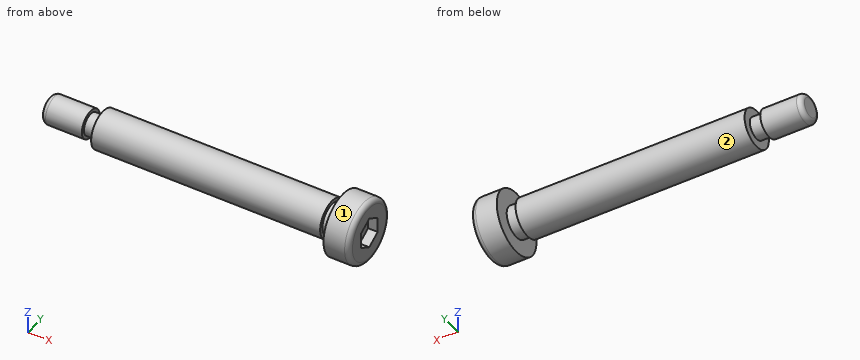
```python
from build123d import *

# Parameters (mm, degrees)
CUT_EXTRUDE1_DEPTH = 2


with BuildPart() as part:
    # Sketch2 → Revolve1 (revolve)
    with BuildSketch(Plane.XY):
        with BuildLine():
            Line((-50, 3.97), (-2.3, 3.97))
            Line((-2.3, 3.97), (-2.3, 3.25))
            Line((-2.3, 3.25), (0, 3.25))
            Line((0, 3.25), (0, 6.5))
            Line((0, 6.5), (4.4, 6.5))
            ThreePointArc((4.4, 6.5), (5.107106781, 6.207106781), (5.4, 5.5))
            Line((5.4, 5.5), (5.4, 0))
            Line((5.4, 0), (-61.15, 0))
            Line((-61.15, 0), (-61.15, 1.925))
            ThreePointArc((-61.15, 1.925), (-60.857106781, 2.632106781), (-60.15, 2.925))
            Line((-60.15, 2.925), (-52.6, 2.925))
            Line((-52.6, 2.925), (-52.6, 2.25))
            Line((-52.6, 2.25), (-50, 2.25))
            Line((-50, 2.25), (-50, 3.97))
        make_face()
    revolve(axis=Axis((-61.15, 0, 0), (1, 0, 0)))

    # Sketch3 → Cut-Extrude1 (cut)
    with BuildSketch(Plane(origin=(5.4, 0, 0), x_dir=(0, 0, -1), z_dir=(1, 0, 0))):
        Polygon((1.58771324, 2.75), (-1.58771324, 2.75), (-3.175426481, 0), (-1.58771324, -2.75), (1.58771324, -2.75), (3.175426481, 0), align=None)
    extrude(amount=-CUT_EXTRUDE1_DEPTH, mode=Mode.SUBTRACT)


solid = part.part
```
CAD build for the part. Positions are in the model's coordinates, mm. Face numbers are marked on the shaded views. A direction names the side the tool comes from. Coordinates: 2 decimals unless noted, no trailing zeros. Loops run counter-clockwise (first coordinate to the right, second up) from the corner with the lowest first, then second, coordinate; pieces in that order, holes last. Notation, with made-up numbers: (-21.75, 54.25) - (-2.75, 54.25) arc R18 cw to (-2.75, 75.25) - close; hole circle Ø4 at (-26, -5). An arc over 180 degrees is marked (long way). Use CSV: the item, a comma, the result in double quotes. Start each with the question number.
Q1. Cut at B-B, the plane x = 1. List the corners of the cut face in (y, z).
Q2. 3-axis set-ups, long thin cutter, end or side, ignore diameter. For the marked faces 1 and 2: which of +Z, -Z, +X, -X, +Y, -Y reach the whole face in a straight line?
Q3. Cut at A-A, the plane z = 0. List the corners of the cut face in (x, y) (3 decimals), then the cut area to 3 significant figures.
Q4. Probe probe 1 along X at (y, z) = (3.75, -0.5); probe 2 along X at (y, z) = (4, 1); probe 3 along X at (y, z) = (-0.5, -1.5). List the from-to ranges inside material, lowest first. Write a range as from..to.
Q5. Drop flat-ended pins along their axis: P1, Ø0.6, axis at x = 4, z = -0.5, coming from the +Y side; P2, Ø4, axis at x = -23.5, y = 5, coming from the +Z side; P3, Ø1.6, axis at y = 1, z = 1, coming from the +X side. Give the stop position or say it passes through.
Here are the results:
1,outline,"circle Ø13 at (0, 0)"
2,face 1,"+X, -X"
2,face 2,"-X"
3,outline,"(-61.15, -1.925) arc R1 ccw to (-60.15, -2.925) - (-52.6, -2.925) - (-52.6, -2.25) - (-50, -2.25) - (-50, -3.97) - (-2.3, -3.97) - (-2.3, -3.25) - (0, -3.25) - (0, -6.5) - (4.4, -6.5) arc R1 ccw to (5.4, -5.5) - (5.4, -2.75) - (3.4, -2.75) - (3.4, 2.75) - (5.4, 2.75) - (5.4, 5.5) arc R1 ccw to (4.4, 6.5) - (0, 6.5) - (0, 3.25) - (-2.3, 3.25) - (-2.3, 3.97) - (-50, 3.97) - (-50, 2.25) - (-52.6, 2.25) - (-52.6, 2.925) - (-60.15, 2.925) arc R1 ccw to (-61.15, 1.925) - close"
3,area,"514 mm2"
4,probe 1,"-50..-2.3, 0..5.4"
4,probe 2,"0..5.4"
4,probe 3,"-61.15..3.4"
5,P1,"y = 6.5"
5,P2,"z = 2.6"
5,P3,"x = 3.4"
